from build123d import *

# Parameters (mm, degrees)
F1_DEPTH = 6.95
F2_R     = 2.5
F3_DEPTH = 40
F6_R     = 3
F7_DEPTH = 10


with BuildPart() as f1:
    # F0 (on Top) → F1 (new body)
    with BuildSketch(Plane.XY):
        with BuildLine():
            Line((-5.050165, -7.449553), (5.050165, -7.449553))
            ThreePointArc((5.050165, -7.449553), (0, 9), (-5.050165, -7.449553))
        make_face()
    extrude(amount=F1_DEPTH)

    # F2 (on face) → F3 (join)
    with BuildSketch(Plane.XZ.offset(7.449553)):
        with Locations((0, 3.475)):
            Circle(F2_R)
    extrude(amount=F3_DEPTH)

    # F4 (on face) → F5 (revolve)
    with BuildSketch(Plane.XZ.offset(47.449553)):
        with BuildLine():
            Line((0, 0.975), (0, -4.025))
            ThreePointArc((0, -4.025), (7.5, 3.475), (0, 10.975))
            Line((0, 10.975), (0, 5.975))
            ThreePointArc((0, 5.975), (1.767767, 5.242767), (2.5, 3.475))
            ThreePointArc((2.5, 3.475), (1.767767, 1.707233), (0, 0.975))
        make_face()
    revolve(axis=Axis((0, -47.449553, 3.475), (0, 0, -1)))

    # F6 (on face) → F7 (cut)
    with BuildSketch(Plane.XY.offset(6.95)):
        with Locations((-3, -3)):
            Circle(F6_R)
    extrude(amount=-F7_DEPTH, mode=Mode.SUBTRACT)


solid = f1.part
Verification items for the finished model (mm, model axes). A direction names the side the tool comes from. Coordinates: 2 decimals unless noted, no trailing zeros. Loops run counter-clockwise (first coordinate to the right, second up) from the corner with the lowest first, then second, coordinate; pieces in that order, holes last. Notation, with made-up numbers: (78.5, 41.5) -> (109.5, 41.5) arc R20 ccw to (109.5, 53.5) -> close; hole circle Ø3 at (87.25, -32). An arc over 180 degrees is marked (long way). Answer as CSV lines item,"result".
1) Cross-section at C-C, the plane z = 2.25. Count the separate pieces of the cut face and the enclosed holes in it, then the cut area to 3 significant figures.
Found:
separate pieces,"1"
enclosed holes,"2"
area,"523 mm2"
2) Cross-section at D-D, the plane y = -14.5. Record the cut outline in (x, z) (3 decimals), then the cut area to 3 significant figures.
Found:
outline,"circle Ø5 at (0, 3.475)"
area,"19.6 mm2"
3) Depth check by flat-ended pin: pin 1 (7.5 mm diameter, centred on x = 2, z = 3, fed in from -Y); pin 2 (10 mm diameter, centred on x = -3.5, y = -39, fed in from +Z) (3 decimals); pin 3 (5 mm diameter, centred on x = 1, y = 1.5, fed in from -Z); pin 4 (6 mm diameter, centred on x = -0.5, y = -41.5, fed in from +Z). Enter the tip coordinate at first touch or a pass-through.
Found:
pin 1,"stops at y = -54.95"
pin 2,"stops at z = 9.725"
pin 3,"stops at z = 0"
pin 4,"stops at z = 10.36"
4) Cross-section at B-B, the plane y = -3. Record the cut outline in (x, z), then the cut area to 3 significant figures.
Found:
outline,"(-8.49, 0) -> (-6, 0) -> (-6, 6.95) -> (-8.49, 6.95) -> close; (0, 0) -> (8.49, 0) -> (8.49, 6.95) -> (0, 6.95) -> close"
area,"76.2 mm2"
5) Thickness scan on L1, parallel to Y at x = -0.5, z = 3.25; L2, parallel to Y at x = -3.25, z = 5.25; L3, parallel to Z at x = -5.5, y = 6. Record the ranges inside material, lowest first. Write a range as from..to.
Found:
L1,"y = -54.93..-49.89, -47.45..-4.66, -1.34..8.99"
L2,"y = -53.97..-40.93, -7.45..-5.99, -0.01..8.39"
L3,"z = 0..6.95"
6) Release check for a two-part mould opening along X. For faces 1 (the cylindrical face through (0, 9, 3)), 2 (the cylindrical face through (-5.4, -4.8, 3.5)), 3 (the flat face through (0, 1, 0)) record: +X half, -X half, draft (parallel to the pull), parting line (faces both ways), or undercut.
Found:
face 1,"parting line"
face 2,"undercut"
face 3,"draft"
7) Tool access check on faces 4 (the cylindrical face through (1.344, -23.684, 5.583)), 5 (the flat face through (0, 1, 6.95)). Record the directions out of +Z, -Z, +X, -X, +Y, -Y that give a thin tool (end or side, any length) a straight path to the whole face; none if there is none.
Found:
face 4,"none"
face 5,"+Z, +X, -X, +Y"
8) Cross-section at A-A, the plane x = 3.75. Record the cut outline in (y, z) (3 decimals).
Found:
outline,"circle Ø12.99 at (-47.45, 3.475); (-7.45, 0) -> (8.182, 0) -> (8.182, 6.95) -> (-7.45, 6.95) -> close"
